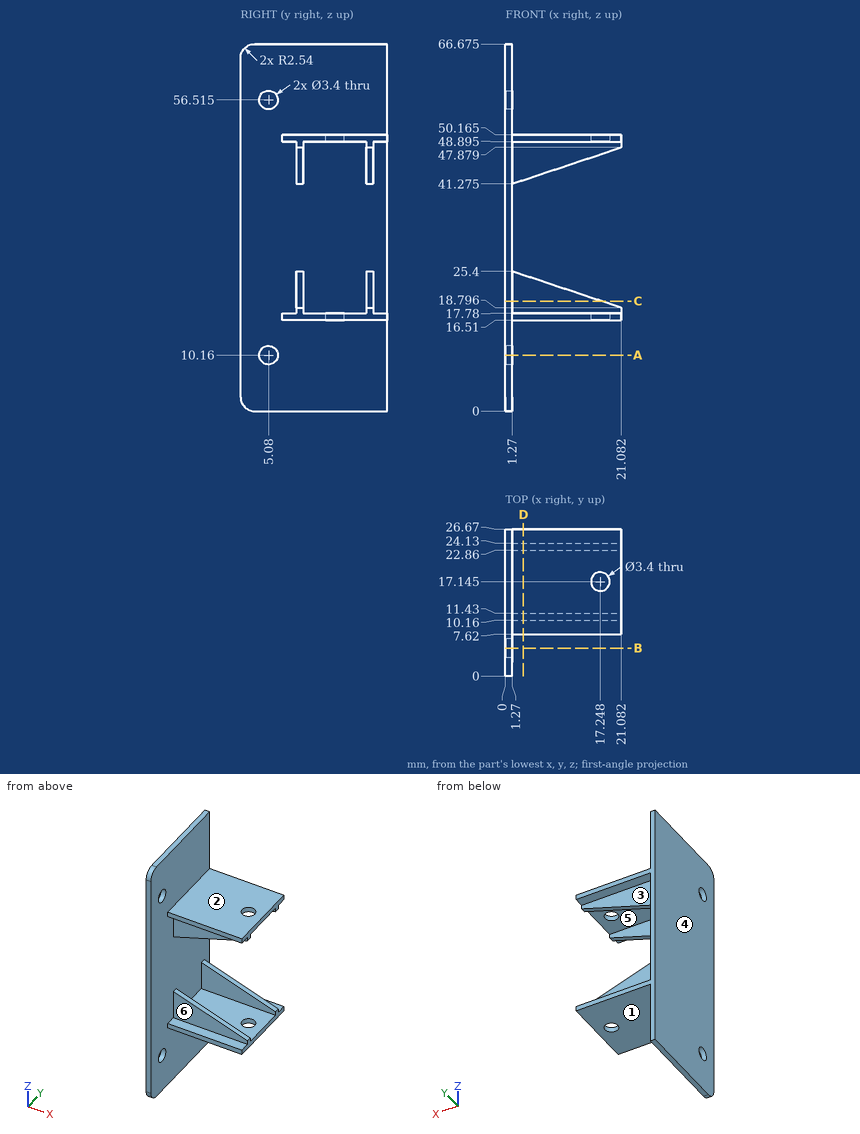
Job drawing, mm, ordinate dimensions from the low corner. One solid piece. A direction names the side the tool comes from. Coordinates: 2 decimals unless noted, no trailing zeros. Write each loop counter-clockwise with the first axis right and the second up, starting at its lowest first coordinate (ties: lowest second). Pieces come first, ordered by that corner, then holes.
Item 1: Slice it at A-A (z = 10.16). Write the cut outline in (x, y).
Item 2: Probe line 1 (Y direction, x = 2.25, z = 23); line 2 (Z direction, x = 11.25, y = 20.25) (1 decimal); line 3 (X direction, y = 8.25, z = 5.5). List the from-to ranges inside material, lowest first.
Item 3: Pin check, flat tips, straight feed: pin 1 (6 mm diameter, centred on x = 13.5, z = 22.5, fed in from +Y); pin 2 (1 mm diameter, centred on x = 10.5, z = 17, fed in from -Y); pin 3 (2 mm diameter, centred on x = 8.5, y = 25, fed in from -Z); pin 4 (2.5 mm diameter, centred on x = 17.25, y = 17.14, fed in from -Z) (3 decimals). Stop position of each tip, or through.
Item 4: Slice it at C-C (z = 20). Write the cut outline in (x, y).
Item 5: Mould opens along Z. For the marked faces 1, 2, 3 and 4 say: released by +Z, released by -Z, zero draft, split by the parting line, or undercut.
Item 6: Slice it at B-B (y = 5.08). Write the cut outline in (x, z) (1 decimal).
Item 7: Slice it at D-D (x = 3.25). Write the cut outline in (y, z) (1 decimal).
Item 8: Which spindle directions (+Z, -Z, +X, -X, +Y, -Y) get a long thin tool onto all of the face, cutting with end or side? Do the marked faces 5 and 6. Say none if no direction does.
Results found:
1. outline: (0, 0) - (1.27, 0) - (1.27, 3.38) - (0, 3.38) - close; (0, 6.78) - (1.27, 6.78) - (1.27, 26.67) - (0, 26.67) - close
2. line 1: y = 10.16 to 11.43, 22.86 to 24.13
2. line 2: z = 16.5 to 17.8, 48.9 to 50.2
2. line 3: x = 0 to 1.27
3. pin 1: stops at y = 24.13
3. pin 2: stops at y = 7.62
3. pin 3: stops at z = 16.51
3. pin 4: passes through
4. outline: (0, 0) - (1.27, 0) - (1.27, 10.16) - (17.47, 10.16) - (17.47, 11.43) - (1.27, 11.43) - (1.27, 22.86) - (17.47, 22.86) - (17.47, 24.13) - (1.27, 24.13) - (1.27, 26.67) - (0, 26.67) - close
5. face 1: released by -Z
5. face 2: released by +Z
5. face 3: undercut
5. face 4: zero draft
6. outline: (0, 0) - (1.3, 0) - (1.3, 8.5) - (0, 8.5) - close; (0, 11.9) - (1.3, 11.9) - (1.3, 54.8) - (0, 54.8) - close; (0, 58.2) - (1.3, 58.2) - (1.3, 66.7) - (0, 66.7) - close
7. outline: (7.6, 16.5) - (26.7, 16.5) - (26.7, 17.8) - (24.1, 17.8) - (24.1, 24.7) - (22.9, 24.7) - (22.9, 17.8) - (11.4, 17.8) - (11.4, 24.7) - (10.2, 24.7) - (10.2, 17.8) - (7.6, 17.8) - close; (7.6, 48.9) - (10.2, 48.9) - (10.2, 41.9) - (11.4, 41.9) - (11.4, 48.9) - (22.9, 48.9) - (22.9, 41.9) - (24.1, 41.9) - (24.1, 48.9) - (26.7, 48.9) - (26.7, 50.2) - (7.6, 50.2) - close
8. face 5: +X
8. face 6: +X, -Y
